Can you work these out from the model? Positions are in its coordinate system, mm. Face numbers are marked on the shaded views. A direction names the side the tool comes from. Give positions to 0.01 mm unless a question says otherwise; leave off trailing zeros. Loops run counter-clockwise (first coordinate to the right, second up) from the corner with the lowest first, then second, coordinate; pieces in that order, holes last. Notation, with made-up numbers: M 32.25,-7.5 L 78.25,-7.5 A20 cw 78.25,-3.5 Z; hole C 49.5,27.5 d6. An arc over 180 degrees is marked long. Use CSV: the item, a comma, the result in double quotes.
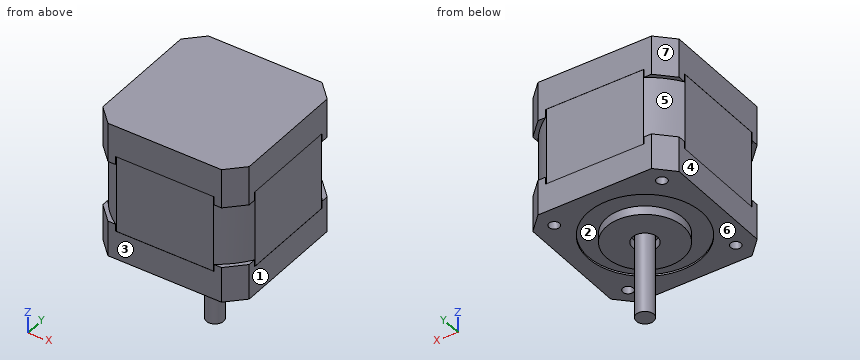
from build123d import *

# Parameters (mm, degrees)
F1_DEPTH      = 11.23
F4_DEPTH      = 10.18
F6_DEPTH      = 2.36
F6_DEPTH_BACK = 19.56
F9_DEPTH      = 21.92
F10_R         = 16.25
F11_DEPTH     = 0.5
F12_R         = 11
F12_R_2       = 3.6
F13_DEPTH     = 2.5
F14_R         = 2.5
F15_DEPTH     = 24.7
F16_R         = 1.5
F17_DEPTH     = 4.5


with BuildPart() as f1:
    # F0 (on Top) → F1 (new body)
    with BuildSketch(Plane.XY):
        Polygon((-16.2600298938, 20.955), (-20.955, 16.2600298938), (-20.955, -16.2600298938), (-16.2600298938, -20.955), (16.2600298938, -20.955), (20.955, -16.2600298938), (20.955, 16.2600298938), (16.2600298938, 20.955), align=None)
    extrude(amount=F1_DEPTH)


with BuildPart() as f4:
    # F3 (on offset) → F4 (new body)
    with BuildSketch(Plane(origin=(0, 0, -17.53), x_dir=(1, 0, 0), z_dir=(0, 0, -1))):
        Polygon((-16.2600298938, 20.955), (-20.955, 16.2600298938), (-20.955, -16.2600298938), (-16.2600298938, -20.955), (16.2600298938, -20.955), (20.955, -16.2600298938), (20.955, 16.2600298938), (16.2600298938, 20.955), align=None)
    extrude(amount=F4_DEPTH)


with BuildPart() as f6_tool:
    # F5 (on face) → F6 (new body, two sides)
    with BuildSketch(Plane(origin=(0, 0, 0), x_dir=(1, 0, 0), z_dir=(0, 0, -1))) as f6_sk:
        with BuildLine():
            Line((20.955, -14.0872451175), (20.955, 14.0872451175))
            ThreePointArc((20.955, 14.0872451175), (17.854446225, 17.854446225), (14.0872451175, 20.955))
            Line((14.0872451175, 20.955), (-14.0872451175, 20.955))
            ThreePointArc((-14.0872451175, 20.955), (-17.854446225, 17.854446225), (-20.955, 14.0872451175))
            Line((-20.955, 14.0872451175), (-20.955, -14.0872451175))
            ThreePointArc((-20.955, -14.0872451175), (-17.854446225, -17.854446225), (-14.0872451175, -20.955))
            Line((-14.0872451175, -20.955), (14.0872451175, -20.955))
            ThreePointArc((14.0872451175, -20.955), (17.854446225, -17.854446225), (20.955, -14.0872451175))
        make_face()
    extrude(amount=-F6_DEPTH)
    extrude(f6_sk.sketch, amount=F6_DEPTH_BACK)


with BuildPart() as f1_1:
    add(f1.part)

    # F6: cut by f6_tool
    add(f6_tool.part, mode=Mode.SUBTRACT)



with BuildPart() as f4_1:
    add(f4.part)

    # F6: cut by f6_tool
    add(f6_tool.part, mode=Mode.SUBTRACT)


with BuildPart() as f1_2:
    add(f1_1.part)

    add(f4_1.part)  # F9 merges F4
    # F8 (on offset) → F9 (join)
    with BuildSketch(Plane.XY.offset(2.36)):
        with BuildLine():
            Line((13.8906263358, 20.93), (-13.8906263358, 20.93))
            ThreePointArc((-13.8906263358, 20.93), (-17.7625223434, 17.7625223434), (-20.93, 13.8906263358))
            Line((-20.93, 13.8906263358), (-20.93, -13.8906263358))
            ThreePointArc((-20.93, -13.8906263358), (-17.7625223434, -17.7625223434), (-13.8906263358, -20.93))
            Line((-13.8906263358, -20.93), (13.8906263358, -20.93))
            ThreePointArc((13.8906263358, -20.93), (17.7625223434, -17.7625223434), (20.93, -13.8906263358))
            Line((20.93, -13.8906263358), (20.93, 13.8906263358))
            ThreePointArc((20.93, 13.8906263358), (17.7625223434, 17.7625223434), (13.8906263358, 20.93))
        make_face()
    extrude(amount=-F9_DEPTH)

    # F10 (on face) → F11 (cut)
    with BuildSketch(Plane(origin=(0, 0, -27.71), x_dir=(1, 0, 0), z_dir=(0, 0, -1))):
        Circle(F10_R)
    extrude(amount=-F11_DEPTH, mode=Mode.SUBTRACT)

    # F12 (on face) → F13 (join)
    with BuildSketch(Plane(origin=(0, 0, -27.21), x_dir=(1, 0, 0), z_dir=(0, 0, -1))):
        Circle(F12_R)
        Circle(F12_R_2, mode=Mode.SUBTRACT)
    extrude(amount=F13_DEPTH)

    # F14 (on face) → F15 (join)
    with BuildSketch(Plane(origin=(0, 0, -27.21), x_dir=(1, 0, 0), z_dir=(0, 0, -1))):
        Circle(F14_R)
    extrude(amount=F15_DEPTH)

    # F16 (on face) → F17 (cut)
    with BuildSketch(Plane(origin=(0, 0, -27.71), x_dir=(1, 0, 0), z_dir=(0, 0, -1))):
        with Locations((15.430398907, -15.3814321037)):
            Circle(F16_R)
        with Locations((-15.568696448, -15.6182594076)):
            Circle(F16_R)
        with Locations((-15.430398907, 15.3814321037)):
            Circle(F16_R)
        with Locations((15.568696448, 15.6182594076)):
            Circle(F16_R)
    extrude(amount=-F17_DEPTH, mode=Mode.SUBTRACT)


solid = f1_2.part
Q1. If we mould it in two halves opening along X, with no side actions, what happens to the marked faces 1, 2, 3 and 4? For each: released by +X, released by -X, zero draft, split by the parting line, or undercut.
Model answer:
face 1,"released by +X"
face 2,"undercut"
face 3,"zero draft"
face 4,"released by -X"
Q2. I'm going to push flat-ended pins straight in: P1, Ø12, axis at x = 10.5, z = -41, coming from the +Y side; P2, Ø2, axis at x = 7, z = -9.5, coming from the +Y side; P3, Ø2.5, axis at x = 16, y = -16, coming from the -Z side; P4, Ø6.5, axis at y = 6, z = -10.5, coming from the +X side. Where does each tip first touch, or does it pass through?
Model answer:
P1,"through"
P2,"y = 20.93"
P3,"z = -27.71"
P4,"x = 20.93"
Q3. I want a section at A-A, the plane x = 0. Please give me the cut outline in (y, z) (3 decimals), then the cut area to 3 significant figures.
Model answer:
outline,"M -20.955,-27.71 L -16.25,-27.71 L -16.25,-27.21 L -11,-27.21 L -11,-29.71 L -3.6,-29.71 L -3.6,-27.21 L -2.5,-27.21 L -2.5,-51.91 L 2.5,-51.91 L 2.5,-27.21 L 3.6,-27.21 L 3.6,-29.71 L 11,-29.71 L 11,-27.21 L 16.25,-27.21 L 16.25,-27.71 L 20.955,-27.71 L 20.955,-19.56 L 20.93,-19.56 L 20.93,2.36 L 20.955,2.36 L 20.955,11.23 L -20.955,11.23 L -20.955,2.36 L -20.93,2.36 L -20.93,-19.56 L -20.955,-19.56 Z"
area,"1,780 mm2"
Q4. For the marked faces 5, 6 and 7, which set-ups out of +Z, -Z, +X, -X, +Y, -Y let a thin tool reach every point of the face, with its end or its side?
Model answer:
face 5,"none"
face 6,"-Z"
face 7,"+Z, -Z, -X, +Y"
Q5. Please list where these lines run through material, in increasing order: L1, parallel to X at y = 0, z = -28; L2, parallel to Y at x = 0, z = -27.65 (3 decimals). Write a range as from..to.
Model answer:
L1,"-11..-3.6, -2.5..2.5, 3.6..11"
L2,"-20.955..-16.25, -11..-3.6, -2.5..2.5, 3.6..11, 16.25..20.955"
Q6. I want a section at B-B, the plane z = -14.5. Please give me the cut outline in (x, y).
Model answer:
outline,"M -20.93,-13.89 A25.12 ccw -13.89,-20.93 L 13.89,-20.93 A25.12 ccw 20.93,-13.89 L 20.93,13.89 A25.12 ccw 13.89,20.93 L -13.89,20.93 A25.12 ccw -20.93,13.89 Z"
